```python
from build123d import *

# Parameters (mm, degrees)
BOSS_EXTRUDE1_DEPTH = 1.5875
SKETCH2_W           = 6.35
SKETCH2_H           = 6.35
BOSS_EXTRUDE3_DEPTH = 6.35
SKETCH2_4_R         = 2.54
BOSS_EXTRUDE4_DEPTH = 12.7
BOSS_EXTRUDE4_TAPER = 1.5
CHAMFER1_SIZE       = 1.27
CUT_EXTRUDE1_DEPTH  = 0.6


with BuildPart() as part:
    # Sketch1 → Boss-Extrude1 (new body)
    with BuildSketch(Plane.XY):
        with BuildLine():
            Line((-10.16, 12.7), (10.16, 12.7))
            ThreePointArc((10.16, 12.7), (11.956051224, 11.956051224), (12.7, 10.16))
            Line((12.7, 10.16), (12.7, -10.16))
            ThreePointArc((12.7, -10.16), (11.956051224, -11.956051224), (10.16, -12.7))
            Line((10.16, -12.7), (-10.16, -12.7))
            ThreePointArc((-10.16, -12.7), (-11.956051224, -11.956051224), (-12.7, -10.16))
            Line((-12.7, -10.16), (-12.7, 10.16))
            ThreePointArc((-12.7, 10.16), (-11.956051224, 11.956051224), (-10.16, 12.7))
        make_face()
    extrude(amount=BOSS_EXTRUDE1_DEPTH)

    # Sketch2 → Boss-Extrude3 (add)
    with BuildSketch(Plane.XY.offset(1.5875)):
        with Locations((0, -9.525)):
            Rectangle(SKETCH2_W, SKETCH2_H)
        with Locations((-9.525, 0)):
            Rectangle(SKETCH2_W, SKETCH2_H)
        with Locations((0, 9.525)):
            Rectangle(SKETCH2_W, SKETCH2_H)
    extrude(amount=BOSS_EXTRUDE3_DEPTH)

    # Sketch2<4> → Boss-Extrude4 (add)
    with BuildSketch(Plane.XY.offset(1.5875)):
        Circle(SKETCH2_4_R)
    extrude(amount=BOSS_EXTRUDE4_DEPTH, taper=BOSS_EXTRUDE4_TAPER)

    # Chamfer1
    chamfer1_edges = [part.edges().sort_by_distance(p)[0] for p in [
        (3.175, -9.525, 7.9375),
        (0, -6.35, 7.9375),
        (-3.175, -9.525, 7.9375),
        (-6.35, 0, 7.9375),
        (-9.525, 3.175, 7.9375),
        (-9.525, -3.175, 7.9375),
        (-3.175, 9.525, 7.9375),
        (0, 6.35, 7.9375),
        (3.175, 9.525, 7.9375),
    ]]
    chamfer(chamfer1_edges, length=CHAMFER1_SIZE)

    # Sketch5 → Cut-Extrude1 (cut)
    with BuildSketch(Plane(origin=(0, 0, 0), x_dir=(-1, 0, 0), z_dir=(0, 0, -1))):
        with BuildLine():
            Line((4.9486325, -0.26640625), (4.80566375, 0.53828125))
            Line((4.80566375, 0.53828125), (7.23847625, 0.971875))
            add(Edge.make_bspline(
                [(7.23847625, 0.971875), (7.265300976, 0.977767208), (7.316553027, 0.98902502), (7.386417313, 1.019177205), (7.445975061, 1.058502989), (7.493162343, 1.108540184), (7.528992616, 1.165738145), (7.550544903, 1.23017609), (7.557529133, 1.300086011), (7.551660972, 1.347437558), (7.5486325, 1.371875)],
                knots=[0, 0, 0, 0, 1.152901184, 2.202764348, 3.180935335, 4.133822457, 5.073078543, 5.997854462, 6.966721939, 8, 8, 8, 8], degree=3))
            add(Edge.make_bspline(
                [(7.5486325, 1.371875), (7.542792734, 1.396646864), (7.531543792, 1.444364066), (7.499884848, 1.509487744), (7.454949308, 1.56317803), (7.398478733, 1.60483656), (7.332490711, 1.634793548), (7.257954774, 1.652000254), (7.175330842, 1.654723907), (7.118865714, 1.646499876), (7.0892575, 1.6421875)],
                knots=[0, 0, 0, 0, 1.012727317, 1.950782296, 2.857509254, 3.77751689, 4.725405478, 5.727859725, 6.808574103, 8, 8, 8, 8], degree=3))
            Line((7.0892575, 1.6421875), (4.68535125, 1.2140625))
            Line((4.68535125, 1.2140625), (4.5423825, 2.0140625))
            Line((4.5423825, 2.0140625), (6.80957, 2.41796875))
            add(Edge.make_bspline(
                [(6.80957, 2.41796875), (6.847301022, 2.424146941), (6.920798591, 2.436181655), (7.028827458, 2.450649053), (7.132077261, 2.459484809), (7.230377946, 2.462125573), (7.323482356, 2.462111249), (7.411390055, 2.455615921), (7.494373236, 2.444838372), (7.572748366, 2.429389837), (7.646448474, 2.408717161), (7.716207008, 2.384988312), (7.781584312, 2.355523785), (7.843339322, 2.322401348), (7.900437373, 2.283618978), (7.954078202, 2.241438319), (8.003198202, 2.194332728), (8.049039105, 2.142989061), (8.091852626, 2.08646838), (8.129838889, 2.022351846), (8.165519605, 1.952395345), (8.198803926, 1.875824466), (8.227849252, 1.79261502), (8.254630893, 1.702985573), (8.278091348, 1.606760444), (8.290616987, 1.539909376), (8.29707, 1.50546875)],
                knots=[0, 0, 0, 0, 1.359771566, 2.6487463, 3.875560241, 5.043152735, 6.145362645, 7.185342953, 8.175634619, 9.120170991, 10.023483318, 10.896369062, 11.738034426, 12.571094417, 13.385408157, 14.189651898, 14.995440776, 15.802293543, 16.635868245, 17.512676209, 18.448819778, 19.4278293, 20.479498143, 21.58131884, 22.753933261, 24, 24, 24, 24], degree=3))
            add(Edge.make_bspline(
                [(8.29707, 1.50546875), (8.305210474, 1.455050803), (8.320925979, 1.357716981), (8.329931619, 1.215241739), (8.328455647, 1.08238611), (8.313760468, 0.959261373), (8.287286964, 0.845690636), (8.249314931, 0.741543137), (8.197917555, 0.647303084), (8.133510725, 0.562431816), (8.055481633, 0.485597873), (7.962511247, 0.415961042), (7.855316021, 0.351113951), (7.732146849, 0.29300798), (7.594525824, 0.238879505), (7.440966494, 0.192076113), (7.272810918, 0.149653692), (7.155016591, 0.127243683), (7.093945, 0.115625)],
                knots=[0, 0, 0, 0, 1.145854088, 2.212116218, 3.200227274, 4.124728484, 4.989683175, 5.812791959, 6.605465325, 7.389991602, 8.19606755, 9.055433262, 9.991834628, 11.003714112, 12.108834738, 13.308838049, 14.604741461, 16, 16, 16, 16], degree=3))
            Line((7.093945, 0.115625), (4.9486325, -0.26640625))
        make_face()
        Polygon((3.922449744, 2.991612413), (3.279480994, 3.486924913), (3.716980994, 5.725987413), (3.506824744, 5.406456163), (2.494324744, 4.091612413), (1.858387244, 4.581456163), (4.016980994, 7.384581163), (4.670105994, 6.881456163), (4.235730994, 4.680674913), (4.487293494, 5.041612413), (5.444324744, 6.284581163), (6.081043494, 5.794737413), align=None)
        Polygon((0.751771392, 4.872631367), (-0.046666108, 4.808568867), (-0.151353608, 6.114037617), (-0.860728608, 6.057006367), (-0.756041108, 4.751537617), (-1.555259858, 4.687475117), (-1.838072358, 8.207787617), (-1.038853608, 8.271850117), (-0.920884858, 6.808568867), (-0.211509858, 6.865600117), (-0.329478608, 8.328881367), (0.468958892, 8.392943867), align=None)
        with BuildLine():
            Line((-4.920123047, 0.595953898), (-4.826373047, -0.216546102))
            Line((-4.826373047, -0.216546102), (-7.281841797, -0.500139852))
            add(Edge.make_bspline(
                [(-7.281841797, -0.500139852), (-7.309101197, -0.504525377), (-7.360946713, -0.512866345), (-7.433457472, -0.537944408), (-7.494816887, -0.575051172), (-7.546014611, -0.621374599), (-7.58371574, -0.677092597), (-7.60964659, -0.739143074), (-7.620413138, -0.808422775), (-7.617655389, -0.855861805), (-7.616216797, -0.880608602)],
                knots=[0, 0, 0, 0, 1.159219096, 2.204755514, 3.2015425, 4.154328068, 5.083365855, 6.006192735, 6.959920939, 8, 8, 8, 8], degree=3))
            add(Edge.make_bspline(
                [(-7.616216797, -0.880608602), (-7.612087451, -0.905893532), (-7.604148383, -0.954506266), (-7.575100674, -1.020839716), (-7.534253977, -1.077316595), (-7.481121861, -1.123145326), (-7.416677768, -1.156966932), (-7.343032738, -1.17758862), (-7.260835581, -1.186561346), (-7.203967434, -1.181637993), (-7.174029297, -1.179046102)],
                knots=[0, 0, 0, 0, 1.017435699, 1.956118989, 2.854725016, 3.774173801, 4.725671501, 5.730437334, 6.805192659, 8, 8, 8, 8], degree=3))
            Line((-7.174029297, -1.179046102), (-4.747466797, -0.898577352))
            Line((-4.747466797, -0.898577352), (-4.653716797, -1.705608602))
            Line((-4.653716797, -1.705608602), (-6.941998047, -1.969671102))
            add(Edge.make_bspline(
                [(-6.941998047, -1.969671102), (-6.979984517, -1.973970995), (-7.054264745, -1.982379176), (-7.163293427, -1.988062587), (-7.26697771, -1.990520486), (-7.365314035, -1.989642819), (-7.458349703, -1.98213365), (-7.546070479, -1.971662701), (-7.628308, -1.956064631), (-7.705372141, -1.935810731), (-7.777531248, -1.910521256), (-7.845471851, -1.881756251), (-7.909354744, -1.849199201), (-7.967768966, -1.810775982), (-8.024153378, -1.77089027), (-8.074289427, -1.724361899), (-8.121150212, -1.674806826), (-8.163586952, -1.620459759), (-8.202165452, -1.560662167), (-8.236382549, -1.494529965), (-8.267543902, -1.42243798), (-8.295950134, -1.344038488), (-8.319549412, -1.258986625), (-8.34078426, -1.167787102), (-8.358911173, -1.070332781), (-8.367350833, -1.002796217), (-8.371685547, -0.968108602)],
                knots=[0, 0, 0, 0, 1.358401368, 2.656271125, 3.878299373, 5.04462664, 6.149164663, 7.193836517, 8.183125754, 9.121533832, 10.023068678, 10.89808339, 11.74255937, 12.566705813, 13.381233575, 14.193707968, 14.992572825, 15.803516984, 16.640452849, 17.518106834, 18.446603811, 19.430292147, 20.479137631, 21.581463121, 22.757809497, 24, 24, 24, 24], degree=3))
            add(Edge.make_bspline(
                [(-8.371685547, -0.968108602), (-8.376692516, -0.917117039), (-8.386333471, -0.818932436), (-8.386759784, -0.675990175), (-8.377418654, -0.543614299), (-8.355773496, -0.421440498), (-8.322080643, -0.309778046), (-8.277818396, -0.20797594), (-8.221146313, -0.116958382), (-8.151436375, -0.036551913), (-8.06887484, 0.035456823), (-7.971669117, 0.099177126), (-7.860478577, 0.157273079), (-7.734332484, 0.208492142), (-7.59306219, 0.252557661), (-7.437233214, 0.290507962), (-7.26667048, 0.322596301), (-7.147559299, 0.337973891), (-7.085748047, 0.345953898)],
                knots=[0, 0, 0, 0, 1.149100472, 2.212600804, 3.203039271, 4.123413217, 4.990373702, 5.81446832, 6.607288663, 7.386227576, 8.193727073, 9.05753109, 9.988014473, 11.004768982, 12.108042928, 13.305595731, 14.601772712, 16, 16, 16, 16], degree=3))
            Line((-7.085748047, 0.345953898), (-4.920123047, 0.595953898))
        make_face()
        Polygon((-4.129712078, -2.712198334), (-3.524243328, -3.249698334), (-4.114868328, -5.448135834), (-3.883618328, -5.143448334), (-2.785180828, -3.905948334), (-2.185962078, -4.437979584), (-4.529712078, -7.077823334), (-5.144555828, -6.531729584), (-4.558618328, -4.371573334), (-4.834399578, -4.712979584), (-5.874243328, -5.884073334), (-6.473462078, -5.352042084), align=None)
        Polygon((-1.040071044, -4.84243991), (-0.240071044, -4.84243991), (-0.240071044, -6.14243991), (0.409928956, -6.14243991), (0.409928956, -4.84243991), (1.209928956, -4.84243991), (1.209928956, -8.34243991), (0.409928956, -8.34243991), (0.409928956, -6.89243991), (-0.240071044, -6.89243991), (-0.240071044, -8.34243991), (-1.040071044, -8.34243991), align=None)
    extrude(amount=-CUT_EXTRUDE1_DEPTH, mode=Mode.SUBTRACT)


solid = part.part
```
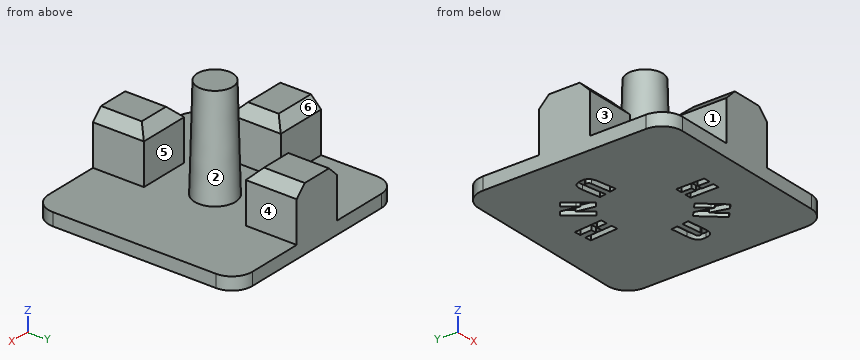
Input: part model. Units: mm. Frame: model coordinates. Face numbers are marked on the shaded views. A direction names the side the tool comes from. Coordinates: 2 decimals unless noted, no trailing zeros. Loops run counter-clockwise (first coordinate to the right, second up) from the corner with the lowest first, then second, coordinate; pieces in that order, holes last. Notation, with made-up numbers: M 7,-34 L 54,-34 A13 cw 54,-19 Z; hole C 3.5,-0.75 d2. An arc over 180 degrees is marked long. Answer in a Markdown table with one row per item.
1. Section B-B, the plane y = 8.75. Output: boundary loops of the cut face in (x, z) (1 decimal).
Response:
| item | result |
|---|---|
| outline | M -12.7,0 L 12.7,0 L 12.7,1.6 L 3.2,1.6 L 3.2,6.7 L 1.9,7.9 L -1.9,7.9 L -3.2,6.7 L -3.2,1.6 L -12.7,1.6 Z |
2. Draft query along Y for the marked faces 1, 2 and 3. Return one class per face: pulls with the +Y half, pulls with the -Y half, needs draft (parallel to the pull), parting line crosses it, or undercut.
Response:
| item | result |
|---|---|
| face 1 | needs draft |
| face 2 | undercut |
| face 3 | pulls with the -Y half |
3. Reachability of the marked faces 4, 5 and 6 from +Z, -Z, +X, -X, +Y, -Y: full face, straight path, thin tool, end or side. Return the list, or none.
Response:
| item | result |
|---|---|
| face 4 | +Z, +X, +Y, -Y |
| face 5 | +Z, +X, -X |
| face 6 | +Z, -X, +Y |
4. Section A-A, the plane z = 4.5. Output: boundary loops of the cut face in (x, y) (3 decimals), then the cut area to 3 significant figures.
Response:
| item | result |
|---|---|
| outline | M -12.7,-3.175 L -6.35,-3.175 L -6.35,3.175 L -12.7,3.175 Z; M -3.175,-12.7 L 3.175,-12.7 L 3.175,-6.35 L -3.175,-6.35 Z; M -3.175,6.35 L 3.175,6.35 L 3.175,12.7 L -3.175,12.7 Z; C 0,0 d4.927 |
| area | 140 mm2 |
5. Material intervals for line 1 (Y direction, x = 3, z = 3); line 2 (Y direction, x = 1.5, z = 2.25); line 3 (Z direction, x = -5, y = 6.25), sorted ascending.
Response:
| item | result |
|---|---|
| line 1 | y = -12.7 to -6.35, 6.35 to 12.7 |
| line 2 | y = -12.7 to -6.35, -2.03 to 2.03, 6.35 to 12.7 |
| line 3 | z = 0 to 1.59 |
6. Section C-C, the plane x = 8.75. Output: boundary loops of the cut face in (y, z).
Response:
| item | result |
|---|---|
| outline | M -12.7,0 L 12.7,0 L 12.7,1.59 L -12.7,1.59 Z |
7. Section D-D, the plane z = 2. Output: boundary loops of the cut face in (x, y) (3 decimals).
Response:
| item | result |
|---|---|
| outline | M -12.7,-3.175 L -6.35,-3.175 L -6.35,3.175 L -12.7,3.175 Z; M -3.175,-12.7 L 3.175,-12.7 L 3.175,-6.35 L -3.175,-6.35 Z; M -3.175,6.35 L 3.175,6.35 L 3.175,12.7 L -3.175,12.7 Z; C 0,0 d5.058 |
8. First-contact query: pin 1 (1.5 mm diameter, centred on y = -9, z = 5, fed in from +X) (3 decimals); pin 2 (3 mm diameter, centred on x = -7.5, z = 6.5, fed in from -Y) (3 decimals); pin 3 (1.5 mm diameter, centred on y = -9, z = 2.5, fed in from -X) (3 decimals). Flat tips, straight axial feed; report the tip coordinate or a pass-through.
Response:
| item | result |
|---|---|
| pin 1 | stops at x = 3.175 |
| pin 2 | stops at y = -3.175 |
| pin 3 | stops at x = -3.175 |
